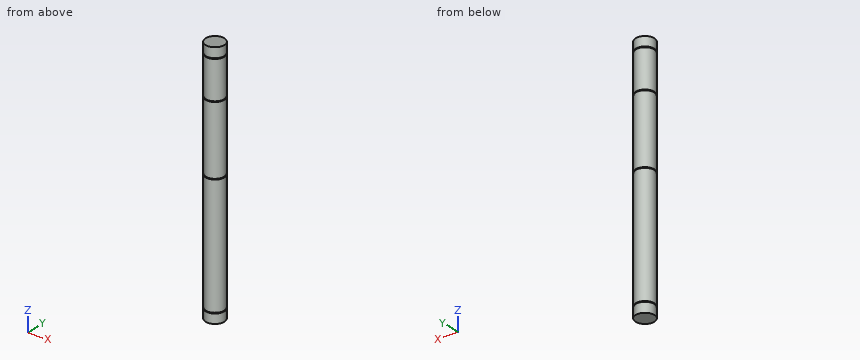
from build123d import *

# Parameters (mm, degrees)
CROQUIS1_R              = 2
SALIENTE_EXTRUIR1_DEPTH = 53
CROQUIS2_W              = 0.25
CROQUIS2_H              = 2


with BuildPart() as part:
    # Croquis1 → Saliente-Extruir1 (new body)
    with BuildSketch(Plane.XY):
        Circle(CROQUIS1_R)
    extrude(amount=SALIENTE_EXTRUIR1_DEPTH)

    # Croquis2 → Cortar-Revolución1 (revolve, cut)
    with BuildSketch(Plane(origin=(0, 0, 0), x_dir=(0, 0, -1), z_dir=(1, 0, 0))):
        with Locations((-50.875, 2.85)):
            Rectangle(CROQUIS2_W, CROQUIS2_H)
        with Locations((-42.625, 2.85)):
            Rectangle(CROQUIS2_W, CROQUIS2_H)
        with Locations((-2.125, 2.85)):
            Rectangle(CROQUIS2_W, CROQUIS2_H)
        with Locations((-27.775, 2.85)):
            Rectangle(CROQUIS2_W, CROQUIS2_H)
    revolve(axis=Axis((0, 0, 0), (0, 0, 1)), mode=Mode.SUBTRACT)


solid = part.part
Geometry check sheet. Reference: the model listing, model coordinates, mm. Round coordinates to 2 decimals unless told otherwise and drop trailing zeros. Loops run counter-clockwise (first coordinate to the right, second up) from the corner with the lowest first, then second, coordinate; pieces in that order, holes last. Notation, with made-up numbers: (88, -15) - (131, -15) arc R20 ccw to (131, 24) - close; hole circle Ø11 at (2.25, 15). An arc over 180 degrees is marked (long way). Answer as CSV lines item,"result".
(1) Depth check by flat-ended pin: pin 1 Ø1 at (x, z) = (1.5, 15) entering from -Y. Enter the tip coordinate at first touch or a pass-through.
Output values:
pin 1,"stops at y = -1.73"
(2) Cross-section at A-A, the plane z = 26. Enter the section's corners in (x, y), and give its area (3 significant figures).
Output values:
outline,"circle Ø4 at (0, 0)"
area,"12.6 mm²"
(3) Material ranges on line 1 along Z through (x, y) = (-1.6, 1.1); line 2 along Y through (x, z) = (-0.15, 39), recorded low to high.
Output values:
line 1,"z = 0 to 2, 2.25 to 27.65, 27.9 to 42.5, 42.75 to 50.75, 51 to 53"
line 2,"y = -1.99 to 1.99"
